```python
from build123d import *

# Parameters (mm, degrees)
ESQUISSE1_W                     = 300
ESQUISSE1_H                     = 190
BOSS_EXTRU_1_DEPTH              = 3
CHANFREIN1_SIZE                 = 10
CONG_1_R                        = 2
ESQUISSE2_R                     = 2.75
ENL_V_MAT_EXTRU_1_DEPTH         = 4
R_P_TITION_LIN_AIRE1_COUNT      = 2
R_P_TITION_LIN_AIRE1_PITCH      = 240
R_P_TITION_LIN_AIRE1_COUNT_DIR2 = 2
R_P_TITION_LIN_AIRE1_PITCH_DIR2 = 160
ESQUISSE3_R                     = 1.6
ENL_V_MAT_EXTRU_2_DEPTH         = 4
R_P_TITION_LIN_AIRE2_COUNT      = 4
R_P_TITION_LIN_AIRE2_PITCH      = 44
ESQUISSE4_R                     = 1.6
ESQUISSE4_R_2                   = 2.75
ENL_V_MAT_EXTRU_3_DEPTH         = 10


with BuildPart() as part:
    # Esquisse1 → Boss.-Extru.1 (new body)
    with BuildSketch(Plane(origin=(0, 0, 0), x_dir=(1, 0, 0), z_dir=(0, 1, 0))):
        Rectangle(ESQUISSE1_W, ESQUISSE1_H)
    extrude(amount=BOSS_EXTRU_1_DEPTH)

    # Chanfrein1
    chanfrein1_edges = [part.edges().sort_by_distance(p)[0] for p in [
        (150, 1.5, 95),
        (-150, 1.5, 95),
        (-150, 1.5, -95),
        (150, 1.5, -95),
    ]]
    chamfer(chanfrein1_edges, length=CHANFREIN1_SIZE)

    # Congé1
    cong_1_edges = [part.edges().sort_by_distance(p)[0] for p in [
        (140, 1.5, 95),
        (-140, 1.5, 95),
        (-150, 1.5, -85),
        (-150, 1.5, 85),
        (150, 1.5, -85),
        (150, 1.5, 85),
        (-140, 1.5, -95),
        (140, 1.5, -95),
    ]]
    fillet(cong_1_edges, radius=CONG_1_R)

    # Esquisse2 → Enlèv. mat.-Extru.1 (cut, through all)
    with BuildSketch(Plane.XZ):
        with Locations((-140, 80)):
            Circle(ESQUISSE2_R)
        with Locations((-100, 80)):
            Circle(ESQUISSE2_R)
    enl_v_mat_extru_1 = extrude(amount=-ENL_V_MAT_EXTRU_1_DEPTH, mode=Mode.SUBTRACT)

    # Répétition linéaire1: Enl_v. mat.-Extru.1 2 × 2
    with Locations(*[(i * R_P_TITION_LIN_AIRE1_PITCH, 0, -j * R_P_TITION_LIN_AIRE1_PITCH_DIR2) for i in range(R_P_TITION_LIN_AIRE1_COUNT) for j in range(R_P_TITION_LIN_AIRE1_COUNT_DIR2) if (i, j) != (0, 0)]):
        add(enl_v_mat_extru_1, mode=Mode.SUBTRACT)

    # Esquisse3 → Enlèv. mat.-Extru.2 (cut, through all)
    with BuildSketch(Plane(origin=(0, 3, 0), x_dir=(1, 0, 0), z_dir=(0, 1, 0))):
        with Locations((-83.75, -80)):
            Circle(ESQUISSE3_R)
        with Locations((-48.25, -80)):
            Circle(ESQUISSE3_R)
        with Locations((-83.75, -11.5)):
            Circle(ESQUISSE3_R)
        with Locations((-48.25, -11.5)):
            Circle(ESQUISSE3_R)
    enl_v_mat_extru_2 = extrude(amount=-ENL_V_MAT_EXTRU_2_DEPTH, mode=Mode.SUBTRACT)

    # Répétition linéaire2: Enlèv. mat.-Extru.2 ×4
    with Locations(*[(i * R_P_TITION_LIN_AIRE2_PITCH, 0, 0) for i in range(1, R_P_TITION_LIN_AIRE2_COUNT)]):
        add(enl_v_mat_extru_2, mode=Mode.SUBTRACT)

    # Esquisse4 → Enlèv. mat.-Extru.3 (cut)
    with BuildSketch(Plane(origin=(0, 3, 0), x_dir=(1, 0, 0), z_dir=(0, 1, 0))):
        with Locations((59.1, 75)):
            Circle(ESQUISSE4_R)
        with Locations((80, 50.6)):
            Circle(ESQUISSE4_R)
        with Locations((100, 80)):
            Circle(ESQUISSE4_R_2)
    extrude(amount=-ENL_V_MAT_EXTRU_3_DEPTH, mode=Mode.SUBTRACT)


solid = part.part
```
The listing builds one solid part. Answer for the finished solid, in the listing's coordinates (mm). Coordinates: 2 decimals unless noted, no trailing zeros. Return JSON: item names as keys, results as strings. Group by question number.
1. Straight lines are drawn through the part: L1, parallel to Z at x = 100, y = 0.8; L2, parallel to X at y = 2.1, z = -50.6; L3, parallel to Z at x = -5.5, y = 2.9. For each, find the intervals that lie inside material, in ascending order.
2. Given pin 1 (3 mm diameter, centred on x = 4.25, z = 11.5, fed in from +Y), flat-ended and moving along its own axis, determine where the tip first touches the part or whether it passes through.
3. Determine the mould class of faces 1 (the flat face through (145, 1, 90)), 2 (the cylindrical face through (-102.747, 1.479, 80.121)), 3 (the flat face through (-2, 3, -1)) for opening direction Z: released by +Z, released by -Z, zero draft, split by the parting line, or undercut.
Ans:
{
 "1": {"L1": "-95 to -82.75, -77.25 to 77.25, 82.75 to 95", "L2": "-150 to 78.4, 81.6 to 150", "L3": "-95 to 10.5, 12.5 to 79, 81 to 95"},
 "2": {"pin 1": "through"},
 "3": {"face 1": "released by +Z", "face 2": "undercut", "face 3": "zero draft"}
}
